Geometry: final body of the model. Coordinates: model frame, mm. Round coordinates to 2 decimals unless told otherwise and drop trailing zeros. Loops run counter-clockwise (first coordinate to the right, second up) from the corner with the lowest first, then second, coordinate; pieces in that order, holes last. Notation, with made-up numbers: (70.5, 13) -> (99.5, 13) arc R25 cw to (99.5, 33) -> close; hole circle Ø2 at (80.5, 40.5). An arc over 180 degrees is marked (long way). Answer in a Markdown table with one row per item.
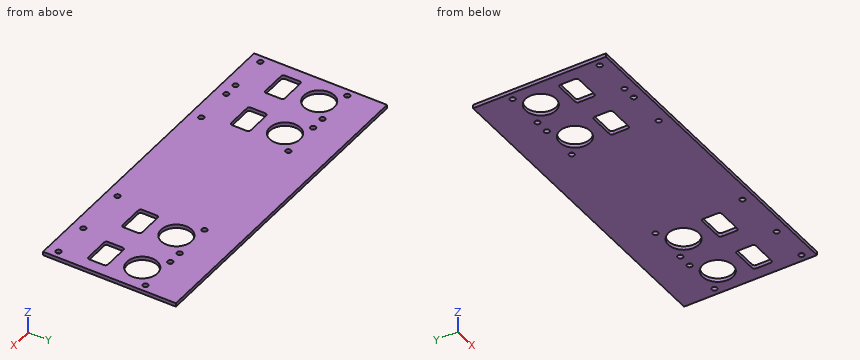
```python
from build123d import *

# Parameters (mm, degrees)
F0_W     = 136
F0_H     = 55
F0_R     = 1.1
F0_R_2   = 6.3
F1_DEPTH = 1.5


with BuildPart() as f1:
    # F0 (on Top) → F1 (new body)
    with BuildSketch(Plane.XY):
        Rectangle(F0_W, F0_H)
        with Locations((-65, -23)):
            Circle(F0_R, mode=Mode.SUBTRACT)
        with Locations((-49, -23)):
            Circle(F0_R, mode=Mode.SUBTRACT)
        with Locations((-43, -23)):
            Circle(F0_R, mode=Mode.SUBTRACT)
        with Locations((-27, -23)):
            Circle(F0_R, mode=Mode.SUBTRACT)
        with BuildLine():
            ThreePointArc((-51, -11.5), (-51.292893, -12.207107), (-52, -12.5))
            Line((-52, -12.5), (-62, -12.5))
            ThreePointArc((-62, -12.5), (-62.707107, -12.207107), (-63, -11.5))
            Line((-63, -11.5), (-63, -5.5))
            ThreePointArc((-63, -5.5), (-62.707107, -4.792893), (-62, -4.5))
            Line((-62, -4.5), (-52, -4.5))
            ThreePointArc((-52, -4.5), (-51.292893, -4.792893), (-51, -5.5))
            Line((-51, -5.5), (-51, -11.5))
        make_face(mode=Mode.SUBTRACT)
        with BuildLine():
            Line((-41, -11.5), (-41, -5.5))
            ThreePointArc((-41, -5.5), (-40.707107, -4.792893), (-40, -4.5))
            Line((-40, -4.5), (-30, -4.5))
            ThreePointArc((-30, -4.5), (-29.292893, -4.792893), (-29, -5.5))
            Line((-29, -5.5), (-29, -11.5))
            ThreePointArc((-29, -11.5), (-29.292893, -12.207107), (-30, -12.5))
            Line((-30, -12.5), (-40, -12.5))
            ThreePointArc((-40, -12.5), (-40.707107, -12.207107), (-41, -11.5))
        make_face(mode=Mode.SUBTRACT)
        with Locations((27, -23)):
            Circle(F0_R, mode=Mode.SUBTRACT)
        with Locations((49, -23)):
            Circle(F0_R, mode=Mode.SUBTRACT)
        with Locations((65, -23)):
            Circle(F0_R, mode=Mode.SUBTRACT)
        with BuildLine():
            ThreePointArc((30, -12.5), (29.292893, -12.207107), (29, -11.5))
            Line((29, -11.5), (29, -5.5))
            ThreePointArc((29, -5.5), (29.292893, -4.792893), (30, -4.5))
            Line((30, -4.5), (40, -4.5))
            ThreePointArc((40, -4.5), (40.707107, -4.792893), (41, -5.5))
            Line((41, -5.5), (41, -11.5))
            ThreePointArc((41, -11.5), (40.707107, -12.207107), (40, -12.5))
            Line((40, -12.5), (30, -12.5))
        make_face(mode=Mode.SUBTRACT)
        with BuildLine():
            Line((52, -4.5), (62, -4.5))
            ThreePointArc((62, -4.5), (62.707107, -4.792893), (63, -5.5))
            Line((63, -5.5), (63, -11.5))
            ThreePointArc((63, -11.5), (62.707107, -12.207107), (62, -12.5))
            Line((62, -12.5), (52, -12.5))
            ThreePointArc((52, -12.5), (51.292893, -12.207107), (51, -11.5))
            Line((51, -11.5), (51, -5.5))
            ThreePointArc((51, -5.5), (51.292893, -4.792893), (52, -4.5))
        make_face(mode=Mode.SUBTRACT)
        with Locations((-57, 6.5)):
            Circle(F0_R_2, mode=Mode.SUBTRACT)
        with Locations((-35, 6.5)):
            Circle(F0_R_2, mode=Mode.SUBTRACT)
        with Locations((-65, 13)):
            Circle(F0_R, mode=Mode.SUBTRACT)
        with Locations((-49, 13)):
            Circle(F0_R, mode=Mode.SUBTRACT)
        with Locations((-43, 13)):
            Circle(F0_R, mode=Mode.SUBTRACT)
        with Locations((-27, 13)):
            Circle(F0_R, mode=Mode.SUBTRACT)
        with Locations((27, 13)):
            Circle(F0_R, mode=Mode.SUBTRACT)
        with Locations((35, 6.5)):
            Circle(F0_R_2, mode=Mode.SUBTRACT)
        with Locations((57, 6.5)):
            Circle(F0_R_2, mode=Mode.SUBTRACT)
        with Locations((43, 13)):
            Circle(F0_R, mode=Mode.SUBTRACT)
        with Locations((49, 13)):
            Circle(F0_R, mode=Mode.SUBTRACT)
        with Locations((65, 13)):
            Circle(F0_R, mode=Mode.SUBTRACT)
    extrude(amount=F1_DEPTH)


solid = f1.part
```
Item 1: Cut plane A-A (x = -57). Output: boundary loops of the cut face in (y, z).
Answer:
| item | result |
|---|---|
| outline | (-27.5, 0) -> (-12.5, 0) -> (-12.5, 1.5) -> (-27.5, 1.5) -> close; (-4.5, 0) -> (0.2, 0) -> (0.2, 1.5) -> (-4.5, 1.5) -> close; (12.8, 0) -> (27.5, 0) -> (27.5, 1.5) -> (12.8, 1.5) -> close |
Item 2: Cut plane D-D (y = 2). Output: boundary loops of the cut face in (x, z), then the cut area to 3 significant figures.
Answer:
| item | result |
|---|---|
| outline | (-68, 0) -> (-61.41, 0) -> (-61.41, 1.5) -> (-68, 1.5) -> close; (-52.59, 0) -> (-39.41, 0) -> (-39.41, 1.5) -> (-52.59, 1.5) -> close; (-30.59, 0) -> (30.59, 0) -> (30.59, 1.5) -> (-30.59, 1.5) -> close; (39.41, 0) -> (52.59, 0) -> (52.59, 1.5) -> (39.41, 1.5) -> close; (61.41, 0) -> (68, 0) -> (68, 1.5) -> (61.41, 1.5) -> close |
| area | 151 mm² |
Item 3: Cut plane C-C (z = 1.1). Count the separate pieces of the cut face and the enclosed holes in it, then the cut area to 3 significant figures.
Answer:
| item | result |
|---|---|
| separate pieces | 1 |
| enclosed holes | 23 |
| area | 6,540 mm² |
Item 4: Line query: probe 1 along X at (y, z) = (-9, 1.35); probe 2 along Y at (x, z) = (-43, 0.7); probe 3 along Y at (x, z) = (57, 0.55). Output: solid intervals per line, ascending. Write a range as [from, to].
Answer:
| item | result |
|---|---|
| probe 1 | x = [-68, -63], [-51, -41], [-29, 29], [41, 51], [63, 68] |
| probe 2 | y = [-27.5, -24.1], [-21.9, 11.9], [14.1, 27.5] |
| probe 3 | y = [-27.5, -12.5], [-4.5, 0.2], [12.8, 27.5] |
Item 5: Cut plane B-B (y = 10). Output: boundary loops of the cut face in (x, z), then the cut area to 3 significant figures.
Answer:
| item | result |
|---|---|
| outline | (-68, 0) -> (-62.24, 0) -> (-62.24, 1.5) -> (-68, 1.5) -> close; (-51.76, 0) -> (-40.24, 0) -> (-40.24, 1.5) -> (-51.76, 1.5) -> close; (-29.76, 0) -> (29.76, 0) -> (29.76, 1.5) -> (-29.76, 1.5) -> close; (40.24, 0) -> (51.76, 0) -> (51.76, 1.5) -> (40.24, 1.5) -> close; (62.24, 0) -> (68, 0) -> (68, 1.5) -> (62.24, 1.5) -> close |
| area | 141 mm² |
